The listing builds one solid part. Answer for the finished solid, in the listing's coordinates (mm). A direction names the side the tool comes from. Round coordinates to 2 decimals unless told otherwise and drop trailing zeros. Order: outer loops, then holes, each group sorted by start corner. A loop starts at its lowest first (then second) coordinate and runs counter-clockwise, first axis right, second up. Notation, with made-up numbers: M -39,47 L -27,47 A29 ccw -27,71 Z; hole C 76,44.5 d11. An arc over 180 degrees is marked long. Put each result on its own line as item: value. Start each with the question number.
1. Consider line 1 (X direction, y = -20, z = 16.5); line 2 (Z direction, x = 4.5, y = -21); line 3 (Z direction, x = 7.25, y = 4). Determine where each line is inside the solid, lowest interval first.
2. Which of the six approach directions +Z, -Z, +X, -X, +Y, -Y give full straight-line access (tool end or side, diameter ignored) to faces 4 (the face through (-7.124, 0.49, 40.982)), 5 (the face through (13.918, -34.43, 58.443)), 6 (the face through (14, -0.46, 56.97)), 7 (the face through (13.545, 34.43, -57.498))?
3. The part is cut by section B-B (z = 23). Give the vertices of the cut face in (x, y), then the cut area to 3 significant figures.
4. Each of these flat-tipped pins is pushed along its axis until it touches: pin 1 Ø10 at (y, z) = (-21.5, 58.5) entering from -X; pin 2 Ø2 at (y, z) = (-7.5, 43) entering from -X; pin 3 Ø8 at (x, y) = (-2, 14.5) entering from -Z; pin 4 Ø12 at (x, z) = (6, -31.5) entering from -Y. Where does it stop, or does it pass through?
5. The part is cut by section A-A (y = -3.5). Give the vertices of the cut face in (x, z).
6. The mould has two halves that part along Z. Classify faces 1 (the face through (-7.5, 0, -1)), 2 (the face through (13.918, 34.43, 58.443)), 3 (the face through (-2.095, -0.49, -55.369)): +Z half, -Z half, draft (parallel to the pull), parting line (faces both ways), or undercut.
from build123d import *

# Parameters (mm, degrees)
F0_W        = 70
F0_H        = 120
F1_DEPTH    = 7.5
F3_DEPTH    = 70
F4_T4_DEPTH = 168.5345436458
F5_T4_DEPTH = 142.4389014281
F6_R        = 2
F7_T1_DEPTH = 89.4016367136
F7_T3_DEPTH = 96.7750960728
F7_T5_DEPTH = 138.4048613392
F7_T7_DEPTH = 129.7242953335


# Not quite as in the source:
# - a fillet or chamfer that OpenCascade refuses, or shapes differently, is made with other operations: its cross-section is extruded or revolved along the edge and cut away or added


with BuildPart() as f1:
    # F0 (on Right) → F1 (new body, symmetric)
    with BuildSketch(Plane.YZ):
        Rectangle(F0_W, F0_H)
    extrude(amount=F1_DEPTH, both=True)

    # F2 (on face) → F3 (join)
    with BuildSketch(Plane.XZ.offset(35)):
        Polygon((6.7201238232, 77.1365826446), (-7.5, 40), (7.5, 40), (21.7201238232, 77.1365826446), align=None)
        Polygon((7.5, -45), (-7.5, -45), (6.7201238232, -71.4156786483), (21.7201238232, -71.4156786483), align=None)
    extrude(amount=-F3_DEPTH)

    # F4: chamfer of 19 x 7.661 on 1 edges, made by hand


with BuildPart() as f4_tool2:
    # F4_s3 → F4_t4 (new body)
    with BuildSketch(Plane.XZ.offset(-84.2672718229)):
        Polygon((0.161, 60), (-7.5, 41), (-7.5, 60), align=None)
    extrude(amount=F4_T4_DEPTH)

    split(bisect_by=Plane(origin=(-19.8989220202, 0, 7.6195792646), x_dir=(0, 1, 0), z_dir=(-0.933876884, 0, 0.3575946945)), keep=Keep.TOP)


with BuildPart() as f1_1:
    add(f1.part)

    # F4_t1: cut F4_tool2
    add(f4_tool2.part, mode=Mode.SUBTRACT)

    # F5: chamfer of 8.076 x 14 on 1 edges, made by hand


with BuildPart() as f5_tool2:
    # F5_s3 → F5_t4 (new body)
    with BuildSketch(Plane.XZ.offset(71.219450714)):
        Polygon((0.576, -60), (-7.5, -46), (-7.5, -60), align=None)
    extrude(amount=-F5_T4_DEPTH)

    split(bisect_by=Plane(origin=(-24.5966117165, 0, -13.2408812545), x_dir=(0, 1, 0), z_dir=(-0.8805226216, 0, -0.4740041274)), keep=Keep.TOP)


with BuildPart() as f1_2:
    add(f1_1.part)

    # F5_t1: cut F5_tool2
    add(f5_tool2.part, mode=Mode.SUBTRACT)

    # F6
    f6_edges = [f1_2.edges().sort_by_distance(p)[0] for p in [
        (14.610062, -35, 58.568291),
        (7.5, -35, -2.5),
        (14.610062, -35, -58.207839),
        (14.610062, 35, -58.207839),
        (7.5, 35, -2.5),
        (14.610062, 35, 58.568291),
        (21.720124, 0, 77.136583),
        (21.720124, 0, -71.415679),
    ]]
    fillet(f6_edges, radius=F6_R)

    # F7: fillet of radius 20 on 4 edges, made by hand

    # F7_s2 → F7_t1 (cut)
    with BuildSketch(Plane.XZ.offset(-44.7008183568)):
        with BuildLine():
            ThreePointArc((-6.0489277422, 44.5987955748), (-7.1338808548, 40.9289668935), (-7.5, 37.1196726573))
            Line((-7.5, 37.1196726573), (-7.9, 37.1196726573))
            Line((-7.9, 37.1196726573), (-7.9, 41.0776065469))
            Line((-7.9, 41.0776065469), (-6.419906297, 44.7483780332))
            Line((-6.419906297, 44.7483780332), (-6.0489277422, 44.5987955748))
        make_face()
    extrude(amount=F7_T1_DEPTH, mode=Mode.SUBTRACT)

    # F7_s4 → F7_t3 (cut)
    with BuildSketch(Plane.XZ.offset(-48.3875480364)):
        with BuildLine():
            ThreePointArc((-7.5, -40.6449807854), (-6.8194736284, -45.8177884102), (-4.8242061277, -50.6385728345))
            Line((-4.8242061277, -50.6385728345), (-5.1706902503, -50.8384446755))
            Line((-5.1706902503, -50.8384446755), (-7.9, -46.1071003843))
            Line((-7.9, -46.1071003843), (-7.9, -40.6449807854))
            Line((-7.9, -40.6449807854), (-7.5, -40.6449807854))
        make_face()
    extrude(amount=F7_T3_DEPTH, mode=Mode.SUBTRACT)

    # F7_s6 → F7_t5 (cut)
    with BuildSketch(Plane.XZ.offset(-69.2024306696)):
        with BuildLine():
            ThreePointArc((18.8126855564, 77.1365826446), (8.4827015625, 73.1912821466), (1.8278807245, 64.3602388931))
            Line((1.8278807245, 64.3602388931), (1.4543299709, 64.5032767709))
            Line((1.4543299709, 64.5032767709), (6.3465730696, 77.2796205224))
            Line((6.3465730696, 77.2796205224), (6.7201238232, 77.5365826446))
            ThreePointArc((6.7201238232, 77.5365826446), (12.7664046898, 77.5365826446), (18.7788308995, 77.5351473974))
            Line((18.7788308995, 77.5351473974), (18.8126855564, 77.1365826446))
        make_face()
    extrude(amount=F7_T5_DEPTH, mode=Mode.SUBTRACT)

    # F7_s8 → F7_t7 (cut)
    with BuildSketch(Plane.XZ.offset(-64.8621476667)):
        with BuildLine():
            ThreePointArc((1.0582113239, -60.8979600281), (8.2849802368, -68.5111251687), (18.3721027929, -71.4156786483))
            Line((18.3721027929, -71.4156786483), (18.3661715736, -71.8156346717))
            ThreePointArc((18.3661715736, -71.8156346717), (12.546113308, -71.8156786483), (6.7201238232, -71.8156786483))
            Line((6.7201238232, -71.8156786483), (6.3679147746, -71.6052802993))
            Line((6.3679147746, -71.6052802993), (0.7060022753, -61.0875616791))
            Line((0.7060022753, -61.0875616791), (1.0582113239, -60.8979600281))
        make_face()
    extrude(amount=F7_T7_DEPTH, mode=Mode.SUBTRACT)


solid = f1_2.part
Resolved:
1. line 1: -7.5 to 7.5
1. line 2: -65.53 to 69.2
1. line 3: -67.84 to 72.18
2. face 4: +Z, -X, +Y, -Y
2. face 5: +X, -Y
2. face 6: +X, +Y, -Y
2. face 7: +X, +Y
3. outline: M -7.5,-35 L 5.5,-35 A2 ccw 7.5,-33 L 7.5,33 A2 ccw 5.5,35 L -7.5,35 Z
3. area: 1,050 mm2
4. pin 1: x = -2.46
4. pin 2: x = -6.9
4. pin 3: z = -62.47
4. pin 4: y = -35
5. outline: M -7.5,-40.64 A20 ccw -4.82,-50.64 L 0.56,-59.97 L 1.06,-60.9 A20 ccw 18.37,-71.42 A2 ccw 20.13,-68.47 L 7.5,-45 L 7.5,40 L 20.68,74.42 A2 ccw 18.81,77.14 A20 ccw 1.83,64.36 L 0.11,59.87 L -6.05,44.6 A20 ccw -7.5,37.12 Z
6. face 1: draft
6. face 2: undercut
6. face 3: -Z half
